Can you work these out from the drawing? Everything is in mm from the part's minimum corner. Coordinates: 2 decimals unless noted, no trailing zeros. Order: outer loops, then holes, each group sorted by start corner. A loop starts at its lowest first (then second) coordinate and runs counter-clockwise, first axis right, second up. Notation, with made-up numbers: M 1,24.5 L 52,24.5 A13 cw 52,39.5 Z; hole C 63,84.5 d6. An arc over 180 degrees is marked long. One line per question, with ' | ' between items. Start each with the question number.
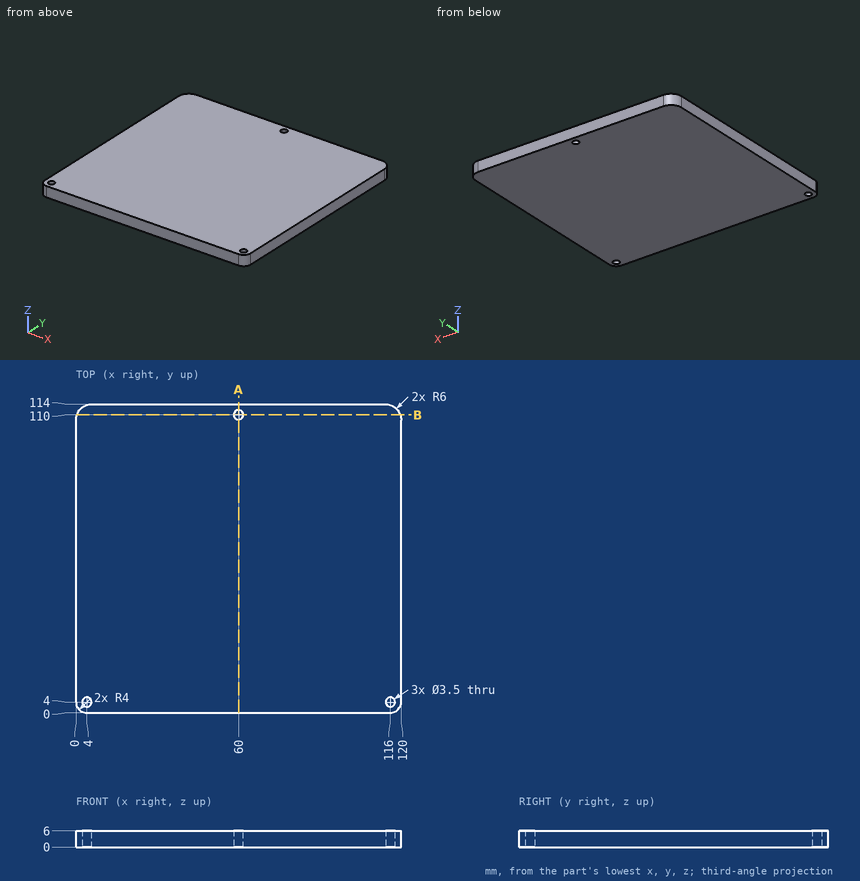
(1) Imagine slicing it at B-B, the plane y = 110. Write out the boundary of the cut face in (x, z), plus the area to 3 significant figures.
(2) If I drill on line 1 along Y through (x, z) = (60, 3.2); line 2 along Y through (x, z) = (116, 3.25); line 3 along X through (y, z) = (110, 2.95), over which ranges is the centre line in solid material (lowest first)? Write a range as from..to.
(3) For P1, Ø3, axis at y = 90, z = 3.5, coming from the -X side; P2, Ø3, axis at x = 4, y = 4, coming from the +Z side, each with a flat end and sliding along its axis, tell me the tip position at first contact or that it passes through.
(4) Imagine slicing it at A-A, the plane x = 60. Write out the boundary of the cut face in (y, z), plus the area to 3 significant figures.
Answers:
1) outline: M 0.34,0 L 58.25,0 L 58.25,6 L 0.34,6 Z; M 61.75,0 L 119.66,0 L 119.66,6 L 61.75,6 Z | area: 695 mm²
2) line 1: 0..108.25, 111.75..114 | line 2: 0..2.25, 5.75..113.66 | line 3: 0.34..58.25, 61.75..119.66
3) P1: x = 0 | P2: through
4) outline: M 0,0 L 108.25,0 L 108.25,6 L 0,6 Z; M 111.75,0 L 114,0 L 114,6 L 111.75,6 Z | area: 663 mm²
